Could you check a few things on this model? Use its own coordinates, in mm. Face numbers are marked on the shaded views. Round coordinates to 2 decimals unless told otherwise and drop trailing zeros. Write each loop counter-clockwise with the first axis right and the second up, starting at its lowest first coordinate (ties: lowest second). Pieces come first, ordered by that corner, then holes. Notation, with made-up numbers: (17, 74.5) -> (59, 74.5) arc R33 ccw to (59, 106.5) -> close; hole circle Ø1 at (13, 48). An arc over 180 degrees is marked (long way). Return JSON: item names as keys, results as strings.
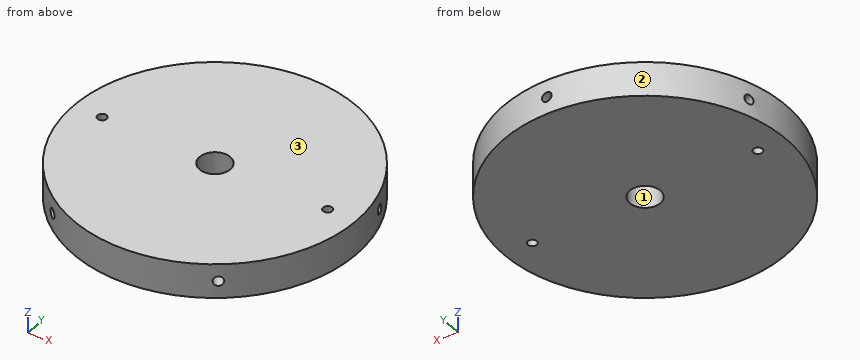
from build123d import *

# Parameters (mm, degrees)
SKETCH1_R                       = 62
BOSS_EXTRUDE1_DEPTH             = 15
M12_CLEARANCE_HOLE1_D           = 13.5
M5_TAPPED_HOLE1_D               = 4.2
M5_TAPPED_HOLE1_DEPTH           = 12.4
M5_TAPPED_HOLE1_TIP             = 1.2618073
M5_TAPPED_HOLE1_ON_FACE_2_D     = 4.2
M5_TAPPED_HOLE1_ON_FACE_2_DEPTH = 12.4
M5_TAPPED_HOLE1_ON_FACE_2_TIP   = 1.2618073
M5_TAPPED_HOLE1_ON_FACE_3_D     = 4.2
M5_TAPPED_HOLE1_ON_FACE_3_DEPTH = 12.4
M5_TAPPED_HOLE1_ON_FACE_3_TIP   = 1.2618073
M5_TAPPED_HOLE1_ON_FACE_4_D     = 4.2
M5_TAPPED_HOLE1_ON_FACE_4_DEPTH = 12.4
M5_TAPPED_HOLE1_ON_FACE_4_TIP   = 1.2618073
M5_TAPPED_HOLE1_ON_FACE_5_D     = 4.2
M5_TAPPED_HOLE1_ON_FACE_5_DEPTH = 12.4
M5_TAPPED_HOLE1_ON_FACE_5_TIP   = 1.2618073
SKETCH12_R                      = 2
CUT_EXTRUDE1_DEPTH              = 32


with BuildPart() as part:
    # Sketch1 → Boss-Extrude1 (new body)
    with BuildSketch(Plane.XY):
        Circle(SKETCH1_R)
    extrude(amount=BOSS_EXTRUDE1_DEPTH)

    # M12 Clearance Hole1 (through all)
    with Locations(Plane(origin=(0, 0, 0), x_dir=(-1, 0, 0), z_dir=(0, 0, -1))):
        with Locations((0, 0)):
            Hole(M12_CLEARANCE_HOLE1_D / 2)

    # M5 Tapped Hole1
    with Locations(Plane(origin=(0, 62, 7.5), x_dir=(1, 0, 0), z_dir=(0, 1, 0))):
        with Locations((0, 0)):
            Hole(M5_TAPPED_HOLE1_D / 2, depth=M5_TAPPED_HOLE1_DEPTH)
            with Locations((0, 0, -(M5_TAPPED_HOLE1_DEPTH + M5_TAPPED_HOLE1_TIP / 2))):  # 118° drill point
                Cone(0, M5_TAPPED_HOLE1_D / 2, M5_TAPPED_HOLE1_TIP, mode=Mode.SUBTRACT)

    # M5 Tapped Hole1 on face 2
    with Locations(Plane(origin=(58.96550401, 19.159053651, 7.5), x_dir=(-0.309016857306, 0.951056560832, 0), z_dir=(0.951056560832, 0.309016857306, 0))):
        with Locations((0, 0)):
            Hole(M5_TAPPED_HOLE1_ON_FACE_2_D / 2, depth=M5_TAPPED_HOLE1_ON_FACE_2_DEPTH)
            with Locations((0, 0, -(M5_TAPPED_HOLE1_ON_FACE_2_DEPTH + M5_TAPPED_HOLE1_ON_FACE_2_TIP / 2))):  # 118° drill point
                Cone(0, M5_TAPPED_HOLE1_ON_FACE_2_D / 2, M5_TAPPED_HOLE1_ON_FACE_2_TIP, mode=Mode.SUBTRACT)

    # M5 Tapped Hole1 on face 3
    with Locations(Plane(origin=(36.442685642, -50.159053651, 7.5), x_dir=(-0.809017116291, -0.58778508449, 0), z_dir=(0.58778508449, -0.809017116291, 0))):
        with Locations((0, 0)):
            Hole(M5_TAPPED_HOLE1_ON_FACE_3_D / 2, depth=M5_TAPPED_HOLE1_ON_FACE_3_DEPTH)
            with Locations((0, 0, -(M5_TAPPED_HOLE1_ON_FACE_3_DEPTH + M5_TAPPED_HOLE1_ON_FACE_3_TIP / 2))):  # 118° drill point
                Cone(0, M5_TAPPED_HOLE1_ON_FACE_3_D / 2, M5_TAPPED_HOLE1_ON_FACE_3_TIP, mode=Mode.SUBTRACT)

    # M5 Tapped Hole1 on face 4
    with Locations(Plane(origin=(-36.442685642, -50.159053651, 7.5), x_dir=(-0.809017116291, 0.58778508449, 0), z_dir=(-0.58778508449, -0.809017116291, 0))):
        with Locations((0, 0)):
            Hole(M5_TAPPED_HOLE1_ON_FACE_4_D / 2, depth=M5_TAPPED_HOLE1_ON_FACE_4_DEPTH)
            with Locations((0, 0, -(M5_TAPPED_HOLE1_ON_FACE_4_DEPTH + M5_TAPPED_HOLE1_ON_FACE_4_TIP / 2))):  # 118° drill point
                Cone(0, M5_TAPPED_HOLE1_ON_FACE_4_D / 2, M5_TAPPED_HOLE1_ON_FACE_4_TIP, mode=Mode.SUBTRACT)

    # M5 Tapped Hole1 on face 5
    with Locations(Plane(origin=(-58.96550401, 19.159053651, 7.5), x_dir=(-0.309016857306, -0.951056560832, 0), z_dir=(-0.951056560832, 0.309016857306, 0))):
        with Locations((0, 0)):
            Hole(M5_TAPPED_HOLE1_ON_FACE_5_D / 2, depth=M5_TAPPED_HOLE1_ON_FACE_5_DEPTH)
            with Locations((0, 0, -(M5_TAPPED_HOLE1_ON_FACE_5_DEPTH + M5_TAPPED_HOLE1_ON_FACE_5_TIP / 2))):  # 118° drill point
                Cone(0, M5_TAPPED_HOLE1_ON_FACE_5_D / 2, M5_TAPPED_HOLE1_ON_FACE_5_TIP, mode=Mode.SUBTRACT)

    # Sketch12 → Cut-Extrude1 (cut)
    with BuildSketch(Plane(origin=(0, 0, 0), x_dir=(-1, 0, 0), z_dir=(0, 0, -1))):
        with Locations((-49.5, 0)):
            Circle(SKETCH12_R)
        with Locations(Location((49.5, 0, 0), (0, 0, 180))):
            Circle(SKETCH12_R)
    extrude(amount=-CUT_EXTRUDE1_DEPTH, mode=Mode.SUBTRACT)


solid = part.part
1) I want a section at B-B, the plane x = 49.5. Count the separate pieces of the cut face and the enclosed holes in it, and give its area (3 significant figures).
Return value:
{"separate pieces": "2", "enclosed holes": "1", "area": "1,050 mm²"}
2) If I drill on probe 1 along Y at (x, z) = (0, 10.5); probe 2 along Z at (x, y) = (0, 58.25); probe 3 along X at (y, z) = (0.5, 9), over which ranges is the centre line in solid material (lowest first)? Write a range as [from, to].
Return value:
{"probe 1": "[-62, -6.75], [6.75, 62]", "probe 2": "[0, 5.4], [9.6, 15]", "probe 3": "[-62, -51.44], [-47.56, -6.73], [6.73, 47.56], [51.44, 62]"}
3) Thinking about a two-plate mould opening in X: for the marked faces 1, 2 and 3, which applies, pulls with the +X half, pulls with the -X half, needs draft (parallel to the pull), parting line crosses it, or undercut?
Return value:
{"face 1": "undercut", "face 2": "parting line crosses it", "face 3": "needs draft"}
4) I want a section at C-C, the plane z = 12. Please give me the cut outline in (x, y), and give its area (3 significant figures).
Return value:
{"outline": "circle Ø124 at (0, 0); hole circle Ø4 at (-49.5, 0); hole circle Ø13.5 at (0, 0); hole circle Ø4 at (49.5, 0)", "area": "11,900 mm²"}
5) I want a section at A-A, the plane y = 0. Please give me the cut outline in (x, z).
Return value:
{"outline": "(-62, 0) -> (-51.5, 0) -> (-51.5, 15) -> (-62, 15) -> close; (-47.5, 0) -> (-6.75, 0) -> (-6.75, 15) -> (-47.5, 15) -> close; (6.75, 0) -> (47.5, 0) -> (47.5, 15) -> (6.75, 15) -> close; (51.5, 0) -> (62, 0) -> (62, 15) -> (51.5, 15) -> close"}
6) I want a section at D-D, the plane x = 22.5. Please give me the cut outline in (y, z), and give its area (3 significant figures).
Return value:
{"outline": "(-57.77, 0) -> (57.77, 0) -> (57.77, 15) -> (-57.77, 15) -> close", "area": "1,730 mm²"}
7) Will these pins go through, and if not, where does the flat tip stop? pin 1 Ø8 at (x, y) = (-5, 21.5) entering from -Z; pin 2 Ø8 at (y, z) = (29, 9.5) entering from -X; pin 3 Ø2.5 at (x, z) = (0, 7.5) entering from +Y; pin 4 Ø6 at (x, z) = (17, 7.5) entering from -Y.
Return value:
{"pin 1": "z = 0", "pin 2": "x = -56.74", "pin 3": "y = 49.09", "pin 4": "y = -60.4"}
